Geometry check sheet. Reference: drawing and pictorial views, mm from the part's lowest x, y, z. A direction names the side the tool comes from. Give positions to 0.01 mm unless a question says otherwise; leave off trailing zeros. Loops run counter-clockwise (first coordinate to the right, second up) from the corner with the lowest first, then second, coordinate; pieces in that order, holes last. Notation, with made-up numbers: (56.5, 54) -> (100.5, 54) arc R21 ccw to (100.5, 85) -> close; hole circle Ø3 at (-25, 81). An arc over 180 degrees is marked (long way). Write each question's results on one line, items separated by ' | '. Start each with the question number.
1. Mould release check, pull along Z, two halves, no side actions. Record for the marked faces 1, 2 and 3: +Z half, -Z half, draft (parallel to the pull), parting line (faces both ways), or undercut.
2. Material ranges on L1, parallel to Z at x = 41, y = 3.9 (3 decimals); L2, parallel to X at y = 4.25, z = 25.5; L3, parallel to X at y = 3.2, z = 24.5, recorded low to high. Write a range as from..to.
3. Cross-section at D-D on z = 25. Record the boundary of the cut face in (x, y).
4. Cross-section at B-B on x = 9. Record the boundary of the cut face in (y, z) (3 decimals).
5. Cross-section at C-C on y = 0.55. Record the boundary of the cut face in (x, z) (3 decimals), and give its area (3 significant figures).
6. Cross-section at A-A on z = 6.5. Record the boundary of the cut face in (x, y), and give its area (3 significant figures).
7. Gauge pin test, flat ends, axial feed: pin 1 Ø1.5 at (x, y) = (44, 1.5) entering from +Z; pin 2 Ø2.5 at (y, z) = (2.5, 6) entering from +X. Record the tip position at first contact, or that the pin passes through.
8. Tool access check on the marked faces 4 and 5. Record the directions out of +Z, -Z, +X, -X, +Y, -Y that give a thin tool (end or side, any length) a straight path to the whole face; none if there is none.
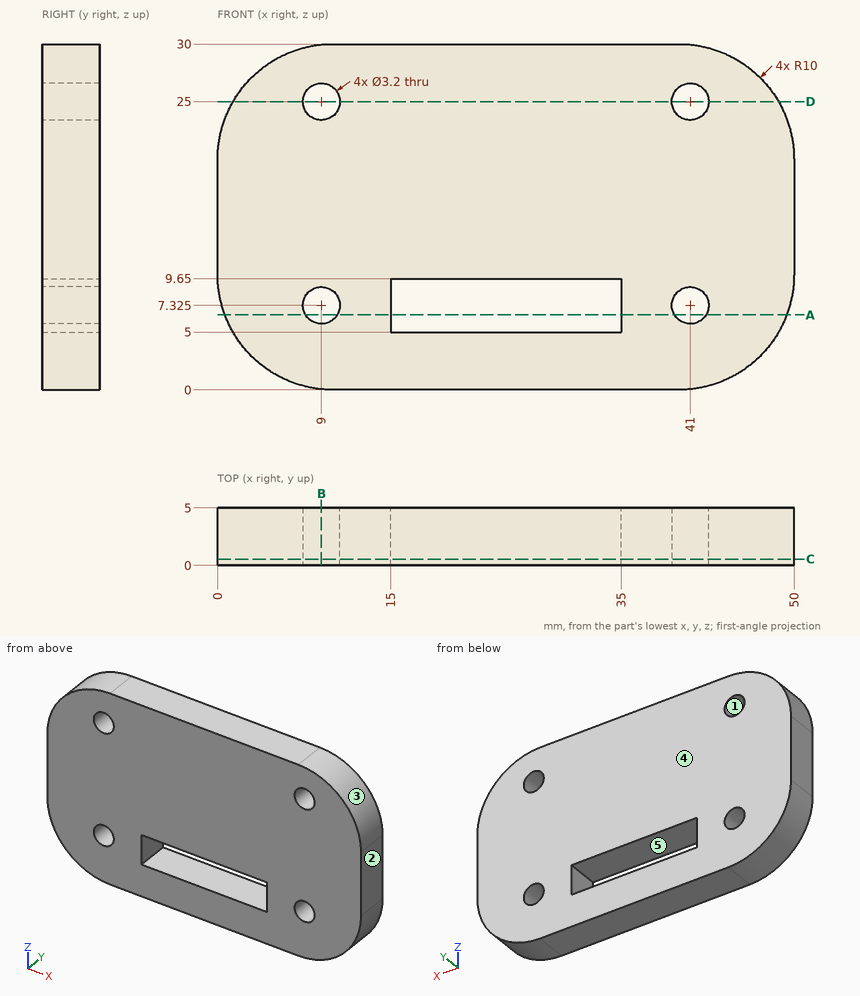
Geometry says:
1) face 1: undercut | face 2: draft | face 3: +Z half
2) L1: 0.05..5.725, 8.925..23.4, 26.6..29.95 | L2: 1.65..7.48, 10.52..39.48, 42.52..48.35 | L3: 1.07..7.48, 10.52..39.48, 42.52..48.93
3) outline: (1.34, 0) -> (7.4, 0) -> (7.4, 5) -> (1.34, 5) -> close; (10.6, 0) -> (39.4, 0) -> (39.4, 5) -> (10.6, 5) -> close; (42.6, 0) -> (48.66, 0) -> (48.66, 5) -> (42.6, 5) -> close
4) outline: (0, 0.05) -> (5, 0.05) -> (5, 5.725) -> (0, 5.725) -> close; (0, 8.925) -> (5, 8.925) -> (5, 23.4) -> (0, 23.4) -> close; (0, 26.6) -> (5, 26.6) -> (5, 29.95) -> (0, 29.95) -> close
5) outline: (0, 10) arc R10 ccw to (10, 0) -> (40, 0) arc R10 ccw to (50, 10) -> (50, 20) arc R10 ccw to (40, 30) -> (10, 30) arc R10 ccw to (0, 20) -> close; hole circle Ø3.2 at (9, 7.325); hole circle Ø3.2 at (9, 25); hole (15, 5) -> (35, 5) -> (35, 9.65) -> (15, 9.65) -> close; hole circle Ø3.2 at (41, 7.325); hole circle Ø3.2 at (41, 25) | area: 1,290 mm^2
6) outline: (0.63, 0) -> (7.63, 0) -> (7.63, 5) -> (0.63, 5) -> close; (10.37, 0) -> (15, 0) -> (15, 5) -> (10.37, 5) -> close; (35, 0) -> (39.63, 0) -> (39.63, 5) -> (35, 5) -> close; (42.37, 0) -> (49.37, 0) -> (49.37, 5) -> (42.37, 5) -> close | area: 116 mm^2
7) pin 1: z = 29.46 | pin 2: x = 49.61
8) face 4: +Z, -Z, +X, -X, +Y | face 5: +Y, -Y
